Read the model definition and answer for the solid it produces. Units are mm, in the model's axes. Face numbers are marked on the shaded views. A direction names the side the tool comes from. Round coordinates to 2 decimals unless told otherwise and drop trailing zeros. Loops run counter-clockwise (first coordinate to the right, second up) from the corner with the lowest first, then second, coordinate; pieces in that order, holes last. Notation, with made-up numbers: M -30.75,43 L -10.75,43 A10 cw -10.75,60 Z; hole C -29.75,2.25 d6. An arc over 180 degrees is marked long. Write each question's results on one line, items separated by ' | '.
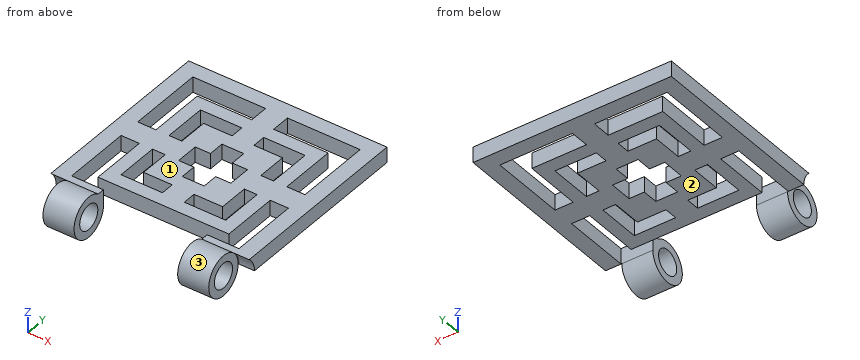
from build123d import *

# Parameters (mm, degrees)
F0_W      = 7.0402130931
F0_H      = 6.0935864692
F0_H_2    = 4.393223295
F0_W_2    = 4.2261239089
F0_H_3    = 7.3185805312
F0_W_3    = 4.3096756666
F0_H_4    = 4.4800786584
F0_H_5    = 4.2855439132
F0_W_4    = 5.8618125553
F0_W_5    = 4.1225401893
F0_W_6    = 4.8947411333
F0_H_6    = 5.0882773987
F1_DEPTH  = 5
F2_R      = 6.5
F2_R_2    = 4
F3_DEPTH  = 63.87
F4_R      = 6.5
F4_R_2    = 4
F5_DEPTH  = 5.25
F6_R      = 6.5
F6_R_2    = 4
F7_DEPTH  = 5.25
F9_R      = 6.5
F9_R_2    = 4
F10_DEPTH = 33.37
F12_DEPTH = 10.25
F14_DEPTH = 10.25


with BuildPart() as f1:
    # F0 (on Top) → F1 (new body)
    with BuildSketch(Plane.XY):
        Polygon((0, 61), (0, 0), (5, 0), (5, 24.3407097344), (5, 31.6592902656), (5, 56), (28.4148934534, 56), (35.4551065466, 56), (58.87, 56), (58.87, 31.6592902656), (58.87, 24.3407097344), (58.87, 0), (63.87, 0), (63.87, 61), align=None)
        Polygon((10.8618125553, 49.9064135308), (10.8618125553, 31.6592902656), (15.0879364642, 31.6592902656), (15.0879364642, 45.5131902358), (28.4148934534, 45.5131902358), (28.4148934534, 49.9064135308), align=None)
        with Locations((31.935, 52.9532067654)):
            Rectangle(F0_W, F0_H)
        Polygon((48.7820635358, 31.6592902656), (53.0081874447, 31.6592902656), (53.0081874447, 49.9064135308), (35.4551065466, 49.9064135308), (35.4551065466, 45.5131902358), (48.7820635358, 45.5131902358), align=None)
        with Locations((31.935, 47.7098018833)):
            Rectangle(F0_W, F0_H_2)
        with Locations((12.9748745097, 28)):
            Rectangle(F0_W_2, F0_H_3)
        Polygon((10.8618125553, 6.0935864692), (28.4148934534, 6.0935864692), (28.4148934534, 10.4868097642), (15.0879364642, 10.4868097642), (15.0879364642, 24.3407097344), (10.8618125553, 24.3407097344), align=None)
        with Locations((31.935, 8.2901981167)):
            Rectangle(F0_W, F0_H_2)
        Polygon((35.4551065466, 10.4868097642), (35.4551065466, 6.0935864692), (53.0081874447, 6.0935864692), (53.0081874447, 24.3407097344), (48.7820635358, 24.3407097344), (48.7820635358, 10.4868097642), align=None)
        with Locations((50.8951254903, 28)):
            Rectangle(F0_W_2, F0_H_3)
        Polygon((40.3498476799, 31.6592902656), (44.6595233465, 31.6592902656), (44.6595233465, 41.2276463227), (35.4551065466, 41.2276463227), (35.4551065466, 36.7475676643), (40.3498476799, 36.7475676643), align=None)
        with Locations((42.5046855132, 28)):
            Rectangle(F0_W_3, F0_H_3)
        Polygon((35.4551065466, 19.2524323357), (35.4551065466, 14.7723536773), (44.6595233465, 14.7723536773), (44.6595233465, 24.3407097344), (40.3498476799, 24.3407097344), (40.3498476799, 19.2524323357), align=None)
        Polygon((19.2104766535, 14.7723536773), (28.4148934534, 14.7723536773), (28.4148934534, 19.2524323357), (23.5201523201, 19.2524323357), (23.5201523201, 24.3407097344), (19.2104766535, 24.3407097344), align=None)
        with Locations((31.935, 17.0123930065)):
            Rectangle(F0_W, F0_H_4)
        with Locations((31.935, 12.6295817207)):
            Rectangle(F0_W, F0_H_5)
        with Locations((21.3653144868, 28)):
            Rectangle(F0_W_3, F0_H_3)
        Polygon((19.2104766535, 41.2276463227), (19.2104766535, 31.6592902656), (23.5201523201, 31.6592902656), (23.5201523201, 36.7475676643), (28.4148934534, 36.7475676643), (28.4148934534, 41.2276463227), align=None)
        with Locations((31.935, 38.9876069935)):
            Rectangle(F0_W, F0_H_4)
        with Locations((55.9390937224, 28)):
            Rectangle(F0_W_4, F0_H_3)
        with Locations((46.7207934411, 28)):
            Rectangle(F0_W_5, F0_H_3)
        with Locations((17.1492065589, 28)):
            Rectangle(F0_W_5, F0_H_3)
        with Locations((7.9309062776, 28)):
            Rectangle(F0_W_4, F0_H_3)
        with Locations((31.935, 43.3704182793)):
            Rectangle(F0_W, F0_H_5)
        with Locations((25.9675228868, 34.2034289649)):
            Rectangle(F0_W_6, F0_H_6)
        with Locations((37.9024771132, 34.2034289649)):
            Rectangle(F0_W_6, F0_H_6)
        with Locations((37.9024771132, 21.7965710351)):
            Rectangle(F0_W_6, F0_H_6)
        with Locations((25.9675228868, 21.7965710351)):
            Rectangle(F0_W_6, F0_H_6)
    extrude(amount=F1_DEPTH)

    # F2 (on face) → F3 (join, through all)
    with BuildSketch(Plane(origin=(0, 0, 0), x_dir=(0, -1, 0), z_dir=(-1, 0, 0))):
        with Locations((4, 0)):
            Circle(F2_R)
        with Locations((4, 0)):
            Circle(F2_R_2, mode=Mode.SUBTRACT)
    extrude(amount=-F3_DEPTH)

    # F4 (on face) → F5 (cut)
    with BuildSketch(Plane.YZ.offset(63.87)):
        with Locations((-4, 0)):
            Circle(F4_R)
        with Locations((-4, 0)):
            Circle(F4_R_2, mode=Mode.SUBTRACT)
    extrude(amount=-F5_DEPTH, mode=Mode.SUBTRACT)

    # F6 (on face) → F7 (cut)
    with BuildSketch(Plane(origin=(0, 0, 0), x_dir=(0, -1, 0), z_dir=(-1, 0, 0))):
        with Locations((4, 0)):
            Circle(F6_R)
        with Locations((4, 0)):
            Circle(F6_R_2, mode=Mode.SUBTRACT)
    extrude(amount=-F7_DEPTH, mode=Mode.SUBTRACT)

    # F9 (on offset) → F10 (cut)
    with BuildSketch(Plane(origin=(15.25, 0, 0), x_dir=(0, -1, 0), z_dir=(-1, 0, 0))):
        with Locations((4, 0)):
            Circle(F9_R)
        with Locations((4, 0)):
            Circle(F9_R_2, mode=Mode.SUBTRACT)
    extrude(amount=-F10_DEPTH, mode=Mode.SUBTRACT)

    # F11 (on face) → F12 (join)
    with BuildSketch(Plane(origin=(58.87, 0, 0), x_dir=(0, -1, 0), z_dir=(-1, 0, 0))):
        with BuildLine():
            ThreePointArc((-2.5, 0), (-1.884153616, 2.7616546168), (-0.1533119315, 5))
            Line((-0.1533119315, 5), (-2.5, 5))
            Line((-2.5, 5), (-2.5, 0))
        make_face()
    extrude(amount=F12_DEPTH)

    # F13 (on face) → F14 (join)
    with BuildSketch(Plane.YZ.offset(5)):
        with BuildLine():
            ThreePointArc((0.1533119315, 5), (1.884153616, 2.7616546168), (2.5, 0))
            Line((2.5, 0), (2.5, 5))
            Line((2.5, 5), (0.1533119315, 5))
        make_face()
    extrude(amount=F14_DEPTH)


solid = f1.part
Item 1: For the marked faces 1, 2 and 3, determine the directions among +Z, -Z, +X, -X, +Y, -Y from which every point of the face is accessible in a straight line to the end or side of a thin tool.
Outcome:
face 1: +Z, +X, -X, +Y | face 2: -Z, +X, -X, +Y | face 3: +X, -X
Item 2: The part is cut by section C-C (x = 46). Determine the outline of the cut face in (y, z), plus the area to 3 significant figures.
Outcome:
outline: M 6.09,0 L 10.49,0 L 10.49,5 L 6.09,5 Z; M 24.34,0 L 31.66,0 L 31.66,5 L 24.34,5 Z; M 45.51,0 L 49.91,0 L 49.91,5 L 45.51,5 Z; M 56,0 L 61,0 L 61,5 L 56,5 Z | area: 106 mm2
Item 3: Flat-ended cylindrical pins translate along their axes: pin 1 (2 mm diameter, centred on x = 24, y = 17, fed in from +Z); pin 2 (5.5 mm diameter, centred on x = 37.5, z = 3, fed in from -Y); pin 3 (6 mm diameter, centred on x = 47, y = 15.5, fed in from -Z). Find the tip coordinate at first contact, or state that the pin passes through.
Outcome:
pin 1: stops at z = 5 | pin 2: stops at y = 6.09 | pin 3: stops at z = 0
Item 4: The part is cut by section A-A (x = 55.5). Determine the outline of the cut face in (y, z), plus the area to 3 significant figures.
Outcome:
outline: M 0.15,5 A6.5 ccw long 2.5,0 L 2.5,5 Z; M 24.34,0 L 31.66,0 L 31.66,5 L 24.34,5 Z; M 56,0 L 61,0 L 61,5 L 56,5 Z; hole C -4,0 d8 | area: 148 mm2
Item 5: Straight lines are drawn through the part: line 1 (X direction, y = 39, z = 4.75); line 2 (Y direction, x = 25, z = 2.5); line 3 (Y direction, x = 46, z = 0.25). For each, find the intervals that lie inside material, in ascending order.
Outcome:
line 1: x = 0 to 5, 10.86 to 15.09, 19.21 to 44.66, 48.78 to 53.01, 58.87 to 63.87 | line 2: y = 6.09 to 10.49, 14.77 to 24.34, 31.66 to 41.23, 45.51 to 49.91, 56 to 61 | line 3: y = 6.09 to 10.49, 24.34 to 31.66, 45.51 to 49.91, 56 to 61
Item 6: The part is cut by section D-D (y = 38.5). Determine the outline of the cut face in (x, z), plus the area to 3 significant figures.
Outcome:
outline: M 0,0 L 5,0 L 5,5 L 0,5 Z; M 10.86,0 L 15.09,0 L 15.09,5 L 10.86,5 Z; M 19.21,0 L 44.66,0 L 44.66,5 L 19.21,5 Z; M 48.78,0 L 53.01,0 L 53.01,5 L 48.78,5 Z; M 58.87,0 L 63.87,0 L 63.87,5 L 58.87,5 Z | area: 220 mm2
Item 7: The part is cut by section B-B (y = 23.5). Determine the outline of the cut face in (x, z), plus the area to 3 significant figures.
Outcome:
outline: M 0,0 L 5,0 L 5,5 L 0,5 Z; M 10.86,0 L 15.09,0 L 15.09,5 L 10.86,5 Z; M 19.21,0 L 28.41,0 L 28.41,5 L 19.21,5 Z; M 35.46,0 L 44.66,0 L 44.66,5 L 35.46,5 Z; M 48.78,0 L 53.01,0 L 53.01,5 L 48.78,5 Z; M 58.87,0 L 63.87,0 L 63.87,5 L 58.87,5 Z | area: 184 mm2
